Geometry check sheet. Reference: the model listing, model coordinates, mm. Face numbers are marked on the shaded views. A direction names the side the tool comes from. Give positions to 0.01 mm unless a question says otherwise; leave off trailing zeros. Write each loop counter-clockwise with the first axis right and the second up, starting at its lowest first coordinate (ties: lowest second). Pieces come first, ordered by that corner, then holes. Notation, with made-up numbers: M 89.5,55.25 L 118.5,55.25 A9 ccw 118.5,65.25 Z; hole C 69,-30 d1. An arc over 180 degrees is marked long. One line per item, written item: value. Start each with the question number.
1. Cross-section at C-C on z = 1.75. Record the cut outline in (x, y).
2. Tool access check on the marked faces 5 and 6. Record the directions out of +Z, -Z, +X, -X, +Y, -Y that give a thin tool (end or side, any length) a straight path to the whole face; none if there is none.
3. Gauge pin test, flat ends, axial feed: pin 1 (1.1 mm diameter, centred on x = 3.5, z = 5.5, fed in from -Y); pin 2 (2.5 mm diameter, centred on y = 18.5, z = 4, fed in from -X); pin 3 (1.5 mm diameter, centred on x = -0.5, z = 5, fed in from -Y); pin 4 (5 mm diameter, centred on x = 1, y = -2.5, fed in from +Z). Record the tip position at first contact, or that the pin passes through.
4. Release check for a two-part mould opening along X. For the marked faces 1, 2, 3 and 4 record: pulls with the +X half, pulls with the -X half, needs draft (parallel to the pull), parting line crosses it, or undercut.
5. Cross-section at D-D on x = 0. Record the cut outline in (y, z), then the cut area to 3 significant figures.
6. Scan lines: line 1 (X direction, y = -10, z = 1); line 2 (Z direction, x = -4.8, y = 1); line 3 (Z direction, x = 6.45, y = 1). Record each from-to range of solid material in increasing order.
7. Cross-section at B-B on y = -9.5. Record the cut outline in (x, z), then the cut area to 3 significant figures.
8. Cross-section at A-A on y = 1. Count the separate pieces of the cut face and the enclosed holes in it, then the cut area to 3 significant figures.
from build123d import *

# Parameters (mm, degrees)
F1_DEPTH       = 10
F3_D           = 2.8
F3_CBORE_D     = 4
F3_CBORE_DEPTH = 6
F4_SIZE        = 0.25


with BuildPart() as f1:
    # F0 (on Top) → F1 (new body)
    with BuildSketch(Plane.XY):
        with BuildLine():
            Line((3.85, -20), (8, -20))
            Line((8, -20), (8, 14.4496737048))
            ThreePointArc((8, 14.4496737048), (0, 22.4496737048), (-8, 14.4496737048))
            Line((-8, 14.4496737048), (-8, -20))
            Line((-8, -20), (-3.85, -20))
            Line((-3.85, -20), (-3.85, -15))
            Line((-3.85, -15), (-2.85, -15))
            Line((-2.85, -15), (-2.85, 14.4496737048))
            ThreePointArc((-2.85, 14.4496737048), (-2.2074806008, 16.252318816), (-0.5696284934, 17.2421678193))
            Line((-0.5696284934, 17.2421678193), (-0.5696284934, 20.1496737048))
            ThreePointArc((-0.5696284934, 20.1496737048), (0, 20.7193021982), (0.5696284934, 20.1496737048))
            Line((0.5696284934, 20.1496737048), (0.5696284934, 17.2421678193))
            ThreePointArc((0.5696284934, 17.2421678193), (2.2074806008, 16.252318816), (2.85, 14.4496737048))
            Line((2.85, 14.4496737048), (2.85, -15))
            Line((2.85, -15), (3.85, -15))
            Line((3.85, -15), (3.85, -20))
        make_face()
    extrude(amount=F1_DEPTH)

    # F3 (through all)
    with Locations(Plane(origin=(-8, 0, 0), x_dir=(0, -1, 0), z_dir=(-1, 0, 0))):
        with Locations((-1, 5)):
            CounterBoreHole(F3_D / 2, F3_CBORE_D / 2, F3_CBORE_DEPTH)

    # F4
    f4_edges = [f1.edges().sort_by_distance(p)[0] for p in [
        (5.925, -20, 0),
        (8, -2.775163, 0),
        (0, 22.449674, 0),
        (-8, -2.775163, 0),
        (-5.925, -20, 0),
        (-3.85, -17.5, 0),
        (-3.35, -15, 0),
        (-2.85, -0.275163, 0),
        (-2.207481, 16.252319, 0),
        (-0.569628, 18.695921, 0),
        (0, 20.719302, 0),
        (0.569628, 18.695921, 0),
        (2.207481, 16.252319, 0),
        (2.85, -0.275163, 0),
        (3.35, -15, 0),
        (3.85, -17.5, 0),
        (5.925, -20, 10),
        (8, -2.775163, 10),
        (0, 22.449674, 10),
        (-8, -2.775163, 10),
        (-5.925, -20, 10),
        (-3.85, -17.5, 10),
        (-3.35, -15, 10),
        (-2.85, -0.275163, 10),
        (-2.207481, 16.252319, 10),
        (-0.569628, 18.695921, 10),
        (0, 20.719302, 10),
        (0.569628, 18.695921, 10),
        (2.207481, 16.252319, 10),
        (2.85, -0.275163, 10),
        (3.35, -15, 10),
        (3.85, -17.5, 10),
        (-8, -20, 5),
        (-3.85, -20, 5),
        (3.85, -20, 5),
        (8, -20, 5),
        (8, 2.4, 5),
        (2.85, 2.4, 5),
        (-8, 3, 5),
        (-2.85, 3, 5),
    ]]
    chamfer(f4_edges, length=F4_SIZE)


solid = f1.part
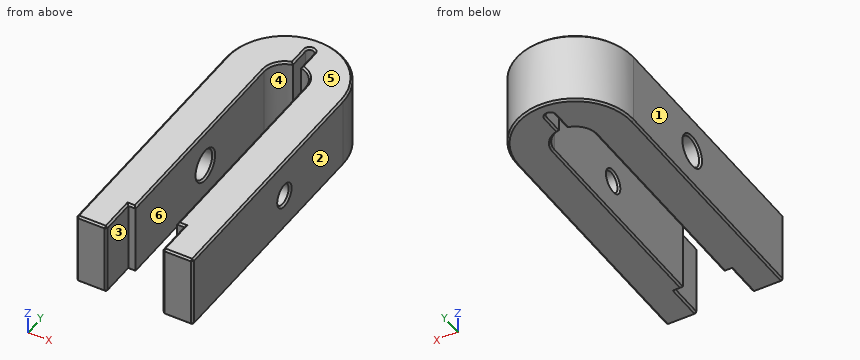
Report:
1. outline: M -8,-19.75 L -7.75,-20 L -4.1,-20 L -3.85,-19.75 L -3.85,-15 L -2.85,-15 L -2.85,14.45 A2.85 cw -0.57,17.24 L -0.57,20.15 A0.57 cw 0.57,20.15 L 0.57,17.24 A2.85 cw 2.85,14.45 L 2.85,-15 L 3.85,-15 L 3.85,-19.75 L 4.1,-20 L 7.75,-20 L 8,-19.75 L 8,14.45 A8 ccw -8,14.45 Z
2. face 5: +Z, +X, -X, +Y, -Y
2. face 6: +Z, -Z, -Y
3. pin 1: stops at y = -19.95
3. pin 2: stops at x = -7.49
3. pin 3: stops at y = 17.01
3. pin 4: stops at z = 10
4. face 1: pulls with the -X half
4. face 2: pulls with the +X half
4. face 3: undercut
4. face 4: undercut
5. outline: M 20.72,0.25 L 20.97,0 L 22.2,0 L 22.45,0.25 L 22.45,9.75 L 22.2,10 L 20.97,10 L 20.72,9.75 Z
5. area: 17.2 mm^2
6. line 1: x = -8 to -2.85, 2.85 to 8
6. line 2: z = 0 to 3, 7 to 10
6. line 3: z = 0 to 3.6, 6.4 to 10
7. outline: M -8,0.25 L -7.75,0 L -3.1,0 L -2.85,0.25 L -2.85,9.75 L -3.1,10 L -7.75,10 L -8,9.75 Z; M 2.85,0.25 L 3.1,0 L 7.75,0 L 8,0.25 L 8,9.75 L 7.75,10 L 3.1,10 L 2.85,9.75 Z
7. area: 103 mm^2
8. separate pieces: 4
8. enclosed holes: 0
8. area: 67.5 mm^2
